Autodesk Inventor part; units mm, degrees
ref_plane "YZ Plane" through (0, 0, 0) normal (1, 0, 0) x (0, 1, 0)
ref_plane "XZ Plane" through (0, 0, 0) normal (0, 1, 0) x (-1, 0, 0)
ref_plane "XY Plane" through (0, 0, 0) normal (0, 0, 1) x (1, 0, 0)
sketch "Skizze1" plane through (0, 0, 0) normal (0, 0, 1) x (1, 0, 0)
  circle A0 centre (0, 0) radius 25
  line L0 (-32.5, 32.5) -> (32.5, 32.5)
  line L1 (32.5, 22.5) -> (32.5, -22.5)
  line L2 (22.5, -32.5) -> (-22.5, -32.5)
  line L3 (-32.5, -22.5) -> (-32.5, 22.5)
  line L4 (-32.5, 32.5) -> (32.5, -32.5) construction
  line L5 (32.5, 32.5) -> (-32.5, -32.5) construction
  circle A1 centre (-25, 25) radius 2.1
  circle A2 centre (25, 25) radius 2.1
  circle A3 centre (-25, -25) radius 2.1
  circle A4 centre (25, -25) radius 2.1
  line L6 (-22.5, 32.5) -> (22.5, 32.5)
  line L7 (32.5, -32.5) -> (-32.5, -32.5)
  line L8 (-32.5, -32.5) -> (-32.5, 32.5)
  line L9 (32.5, 32.5) -> (32.5, -32.5)
  arc A5 (-22.5, 32.5) -> (-32.5, 22.5) centre (-22.5, 22.5) ccw
  arc A6 (-32.5, -22.5) -> (-22.5, -32.5) centre (-22.5, -22.5) ccw
  arc A7 (22.5, -32.5) -> (32.5, -22.5) centre (22.5, -22.5) ccw
  arc A8 (32.5, 22.5) -> (22.5, 32.5) centre (22.5, 22.5) ccw
  dimension "d0" = 50
  dimension "d1" = 65
  dimension "d2" = 65
  dimension "d5" = 25
  dimension "d6" = 25
  dimension "d7" = 4.2
  dimension "d10" = 50
  dimension "d13" = 50
  dimension "d16" = 10
extrude "Extrusion1" add sketch "Skizze1" along normal blind 5 contours L0 A8 L1 A7 L2 A6 L3 A5
sketch "Skizze2" plane through (0, 0, 5) normal (0, 0, 1) x (1, 0, 0)
  circle A0 centre (-25, 25) radius 2.1
  circle A1 centre (-25, 25) radius 3.525
  circle A2 centre (25, 25) radius 2.1
  circle A3 centre (25, 25) radius 3.525
  circle A4 centre (-25, -25) radius 2.1
  circle A5 centre (-25, -25) radius 3.525
  circle A6 centre (25, -25) radius 2.1
  circle A7 centre (25, -25) radius 3.525
  point P0 (0, 0)
  dimension "d17" = 7.05
  dimension "d18" = 7.05
  dimension "d19" = 7.05
  dimension "d20" = 7.05
extrude "Extrusion2" cut sketch "Skizze2" against normal blind 3.2
chamfer "Fase1" distance 1 angle 45 9 edges at (-25, 0, 5) (0, -32.5, 5) (29.5711, -29.5711, 5) (32.5, 0, 5) (29.5711, 29.5711, 5) (0, 32.5, 5) (-29.5711, 29.5711, 5) (-32.5, 0, 5) (-29.5711, -29.5711, 5)
chamfer "Fase2" distance 0.5 angle 45 8 edges at (0, 32.5, 0) (-29.5711, 29.5711, 0) (-32.5, 0, 0) (-29.5711, -29.5711, 0) (0, -32.5, 0) (29.5711, -29.5711, 0) (32.5, 0, 0) (29.5711, 29.5711, 0)
properties part number "StageInsert_FoilHolder_Part1"
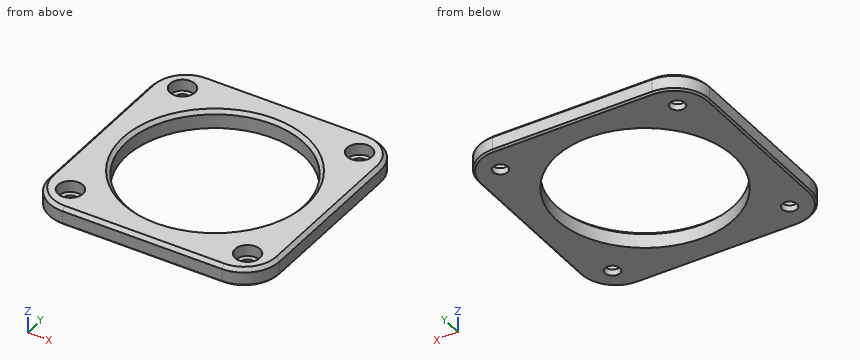
Source: CAD feature listing. Evaluate the final solid. Frame: model axes, mm. Give positions to 0.01 mm unless a question says otherwise; leave off trailing zeros. Write each loop counter-clockwise with the first axis right and the second up, starting at its lowest first coordinate (ties: lowest second). Pieces come first, ordered by that corner, then holes. Notation, with made-up numbers: (60.25, 63) - (66.25, 63) arc R5 ccw to (66.25, 72) - close; hole circle Ø6 at (20, 32.5). An arc over 180 degrees is marked (long way). Write item = value, one per line. Start each with the question number.
Q1. Pin query (flat end, axial travel): pin 1 Ø2 at (x, y) = (-25, -24) entering from +Z; pin 2 Ø3.5 at (x, y) = (25, 25.5) entering from +Z. Return the tip coordinate at first contact, or that it passes through.
Q2. Material intervals for probe 1 along Y at (x, z) = (0, 1.5); probe 2 along X at (y, z) = (25.5, 3.45); probe 3 along X at (y, z) = (6, 3.9), sorted ascending.
Q3. Cut plane A-A, the plane y = 0. Return loops of the section in (x, z).
Q4. Cut plane C-C, the plane z = 3.2. Return loops of the section in (x, y) (3 decimals).
Computed values:
q1.pin_1 = through
q1.pin_2 = 1.8
q2.probe_1 = -32.5 to -25, 25 to 32.5
q2.probe_2 = -32.04 to -28.49, -21.51 to 21.51, 28.49 to 32.04
q2.probe_3 = -32.5 to -24.27, 24.27 to 32.5
q3.outline = (-32.5, 0.5) - (-32, 0) - (-25, 0) - (-25, 4) - (-26, 5) - (-31.5, 5) - (-32.5, 4) - close; (25, 0) - (32, 0) - (32.5, 0.5) - (32.5, 4) - (31.5, 5) - (26, 5) - (25, 4) - close
q4.outline = (-32.5, -22.5) arc R10 ccw to (-22.5, -32.5) - (22.5, -32.5) arc R10 ccw to (32.5, -22.5) - (32.5, 22.5) arc R10 ccw to (22.5, 32.5) - (-22.5, 32.5) arc R10 ccw to (-32.5, 22.5) - close; hole circle Ø7.05 at (-25, -25); hole circle Ø7.05 at (-25, 25); hole circle Ø50 at (0, 0); hole circle Ø7.05 at (25, -25); hole circle Ø7.05 at (25, 25)
